from build123d import *

# Parameters (mm, degrees)
BOSS_EXTRUDE1_DEPTH = 381
CUT_EXTRUDE1_REACH  = 27.4
SKETCH2_R           = 3.429


with BuildPart() as part:
    # Sketch1 → Boss-Extrude1 (new body)
    with BuildSketch(Plane(origin=(0, 0, 0), x_dir=(0, 0, -1), z_dir=(1, 0, 0))):
        Polygon((0, 0), (25.4, 0), (25.4, 3.175), (3.175, 3.175), (3.175, 25.4), (0, 25.4), align=None)
    extrude(amount=BOSS_EXTRUDE1_DEPTH)

    # Sketch2 → Cut-Extrude1 (cut, up to next)
    with BuildSketch(Plane.XZ, mode=Mode.PRIVATE) as cut_extrude1_sk1:
        with Locations((73.66, -12.7)):
            Circle(SKETCH2_R)
    cut_extrude1_tool1 = extrude(cut_extrude1_sk1.sketch, amount=-CUT_EXTRUDE1_REACH, mode=Mode.PRIVATE) & part.part
    add(cut_extrude1_tool1.solids().sort_by_distance((73.66, 0, -12.7))[0], mode=Mode.SUBTRACT)
    # Sketch2 → Cut-Extrude1 (cut, up to next)
    with BuildSketch(Plane.XZ, mode=Mode.PRIVATE) as cut_extrude1_sk2:
        with Locations((368.3, -12.7)):
            Circle(SKETCH2_R)
    cut_extrude1_tool2 = extrude(cut_extrude1_sk2.sketch, amount=-CUT_EXTRUDE1_REACH, mode=Mode.PRIVATE) & part.part
    add(cut_extrude1_tool2.solids().sort_by_distance((368.3, 0, -12.7))[0], mode=Mode.SUBTRACT)
    # Sketch2 → Cut-Extrude1 (cut, up to next)
    with BuildSketch(Plane.XZ, mode=Mode.PRIVATE) as cut_extrude1_sk3:
        with Locations((19.05, -12.7)):
            Circle(SKETCH2_R)
    cut_extrude1_tool3 = extrude(cut_extrude1_sk3.sketch, amount=-CUT_EXTRUDE1_REACH, mode=Mode.PRIVATE) & part.part
    add(cut_extrude1_tool3.solids().sort_by_distance((19.05, 0, -12.7))[0], mode=Mode.SUBTRACT)


solid = part.part
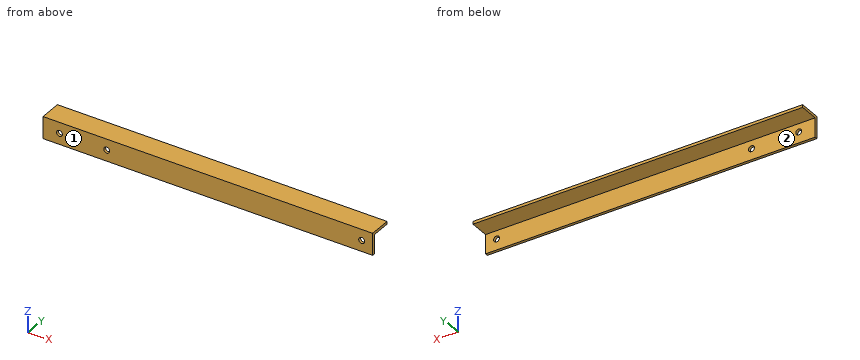
Input: part model. Units: mm. Frame: model coordinates. Face numbers are marked on the shaded views. A direction names the side the tool comes from. Round coordinates to 2 decimals unless told otherwise and drop trailing zeros. Order: outer loops, then holes, each group sorted by start corner. A loop starts at its lowest first (then second) coordinate and runs counter-clockwise, first axis right, second up.
1. Cut plane A-A, the plane x = 73.66. Output: boundary loops of the cut face in (y, z) (3 decimals).
The answers:
outline: (0, -25.4) - (3.175, -25.4) - (3.175, -16.129) - (0, -16.129) - close; (0, -9.271) - (3.175, -9.271) - (3.175, -3.175) - (25.4, -3.175) - (25.4, 0) - (0, 0) - close
2. Pin query (flat end, axial travel): P1, Ø10, axis at x = 300, y = 3.5, coming from the +Z side; P2, Ø11, axis at x = 73.66, z = -12.7, coming from the +Y side (3 decimals); P3, Ø1, axis at x = 174, y = 18.5, coming from the -Z side (3 decimals). Return the tip coordinate at first contact, or that it passes through.
The answers:
P1: stops at z = 0
P2: stops at y = 3.175
P3: stops at z = -3.175
3. Material intervals for line 1 (Z direction, x = 368.3, y = 1.25); line 2 (Z direction, x = 252, y = 10.5) (3 decimals); line 3 (Y direction, x = 155, z = -23.75) (3 decimals), sorted ascending.
The answers:
line 1: z = -25.4 to -16.13, -9.27 to 0
line 2: z = -3.175 to 0
line 3: y = 0 to 3.175
4. Set-up query: the marked faces 1 and 2. Return all of +Z, -Z, +X, -X, +Y, -Y with unobstructed straight access to the full face (end or side cutting, diameter ignored); none if empty.
The answers:
face 1: +Z, -Z, +X, -X, -Y
face 2: -Z, +X, -X, +Y
5. Cut plane C-C, the plane x = 185. Output: boundary loops of the cut face in (y, z) (3 decimals).
The answers:
outline: (0, -25.4) - (3.175, -25.4) - (3.175, -3.175) - (25.4, -3.175) - (25.4, 0) - (0, 0) - close
6. Cut plane B-B, the plane z = -12.7. Output: boundary loops of the cut face in (x, y) (3 decimals).
The answers:
outline: (0, 0) - (15.621, 0) - (15.621, 3.175) - (0, 3.175) - close; (22.479, 0) - (70.231, 0) - (70.231, 3.175) - (22.479, 3.175) - close; (77.089, 0) - (364.871, 0) - (364.871, 3.175) - (77.089, 3.175) - close; (371.729, 0) - (381, 0) - (381, 3.175) - (371.729, 3.175) - close
7. Cut plane D-D, the plane y = 17.5. Output: boundary loops of the cut face in (x, z) (3 decimals).
The answers:
outline: (0, -3.175) - (381, -3.175) - (381, 0) - (0, 0) - close
